Part model, mm, in its own coordinate system. Face numbers are marked on the shaded views. A direction names the side the tool comes from. Round coordinates to 2 decimals unless told otherwise and drop trailing zeros. Loops run counter-clockwise (first coordinate to the right, second up) from the corner with the lowest first, then second, coordinate; pieces in that order, holes last.
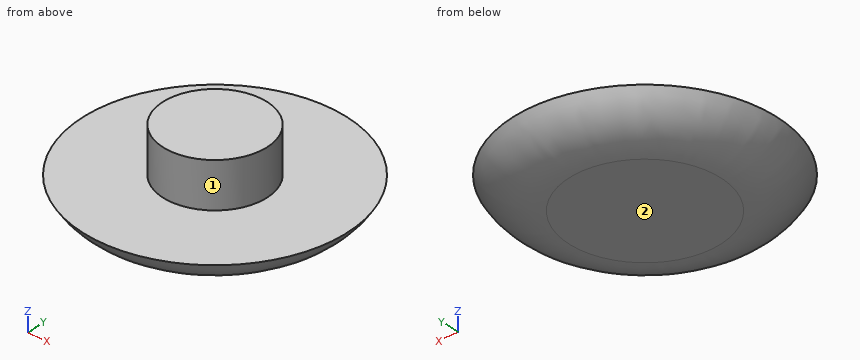
from build123d import *

# Parameters (mm, degrees)
F0_R     = 10.16
F1_DEPTH = 2.5
F2_R     = 4
F3_DEPTH = 3.5


# Not quite as in the source:
# - a fillet or chamfer that OpenCascade refuses, or shapes differently, is made with other operations: its cross-section is extruded or revolved along the edge and cut away or added


with BuildPart() as f1:
    # F0 (on Top) → F1 (new body)
    with BuildSketch(Plane.XY):
        Circle(F0_R)
    extrude(amount=F1_DEPTH)

    # F2 (on face) → F3 (join)
    with BuildSketch(Plane.XY.offset(2.5)):
        Circle(F2_R)
    extrude(amount=F3_DEPTH)

    # F4: fillet of radius 5 on 1 edges, made by hand

    # F4_s1 → F4_t2 (revolve, cut)
    with BuildSketch(Plane.XZ):
        with BuildLine():
            ThreePointArc((10.16, 2.5), (8.3298729811, 0.6698729811), (5.8298729811, 0))
            Line((5.8298729811, 0), (10.16, 0))
            Line((10.16, 0), (10.16, 2.5))
        make_face()
    revolve(axis=Axis((0, 0, 0), (0, 0, 1)), mode=Mode.SUBTRACT)

    # F5: F1 across plane


with BuildPart() as f1_1:
    add(f1.part)
    add(f1.part.mirror(Plane.XZ))


solid = f1_1.part
1) Slice it at C-C, the plane z = 5.5. Give the cut face in (x, y).
Values:
outline: circle Ø8 at (0, 0)
2) Slice it at A-A, the plane x = 0. Give the cut face in (y, z).
Values:
outline: (-10.16, 2.5) arc R5 ccw to (-5.83, 0) - (5.83, 0) arc R5 ccw to (10.16, 2.5) - (4, 2.5) - (4, 6) - (-4, 6) - (-4, 2.5) - close
3) Tool access for the marked faces 1 and 2: list every direction of +Z, -Z, +X, -X, +Y, -Y with a clear straight run to the whole face (end or side of a thin tool).
Values:
face 1: +Z
face 2: -Z, +X, -X, +Y, -Y
4) Wall check: line 1 along Z through (x, y) = (-5.5, 1); line 2 along Z through (x, y) = (-8, -2); line 3 along X through (y, z) = (2, 3.5). Give the ranges that are in metal, low to high.
Values:
line 1: z = 0 to 2.5
line 2: z = 0.62 to 2.5
line 3: x = -3.46 to 3.46
5) Slice it at D-D, the plane z = 1.5. Give the cut face in (x, y).
Values:
outline: circle Ø18.8 at (0, 0)
6) Drop flat-ended pins along their axis: pin 1 Ø2 at (x, y) = (-3, 7) entering from -Z; pin 2 Ø5 at (x, y) = (-5, -3) entering from +Z; pin 3 Ø1.5 at (x, z) = (-3.5, 2) entering from -Y. Give the stop position or say it passes through.
Values:
pin 1: stops at z = 0.06
pin 2: stops at z = 6
pin 3: stops at y = -9.73
